Verification items for the finished model (mm, model axes). Face numbers are marked on the shaded views. A direction names the side the tool comes from. Give positions to 0.01 mm unless a question says otherwise; leave off trailing zeros. Write each loop counter-clockwise with the first axis right and the second up, starting at its lowest first coordinate (ties: lowest second). Pieces come first, ordered by that corner, then holes. Notation, with made-up numbers: (71, 51) -> (101, 51) arc R27 ccw to (101, 82) -> close; hole circle Ø4 at (62.25, 4.25). An arc over 180 degrees is marked (long way). Write item = value, one per line.
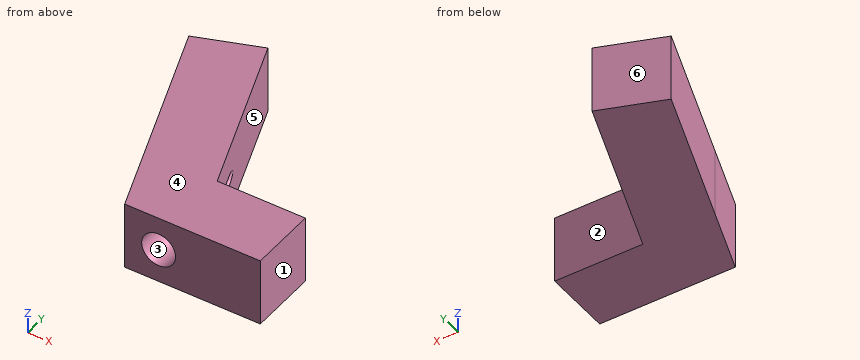
from build123d import *

# Parameters (mm, degrees)
BOSS_EXTRUDE1_DEPTH = 25.4
SKETCH3_R           = 6.35
CUT_EXTRUDE1_DEPTH  = 15.875
SKETCH4_R           = 2.0955
CUT_EXTRUDE2_DEPTH  = 98.893788925


with BuildPart() as part:
    # Sketch1 → Boss-Extrude1 (new body)
    with BuildSketch(Plane.XY):
        Polygon((0, 0), (-19.950187023, 54.81268836), (3.918005545, 63.5), (27.030115421, 0), (60.04484395, 0), (60.04484395, -25.4), (9.24484395, -25.4), align=None)
    extrude(amount=BOSS_EXTRUDE1_DEPTH)

    # Sketch3 → Cut-Extrude1 (cut)
    with BuildSketch(Plane.XZ.offset(25.4)):
        with Locations(Location((21.94484395, 12.7, 0), (0, 0, 270))):
            Circle(SKETCH3_R)
    extrude(amount=-CUT_EXTRUDE1_DEPTH, mode=Mode.SUBTRACT)

    # Sketch4 → Cut-Extrude2 (cut, through all)
    with BuildSketch(Plane.XZ.offset(9.525)):
        with Locations(Location((21.94484395, 12.7, 0), (0, 0, 270))):
            Circle(SKETCH4_R)
    extrude(amount=-CUT_EXTRUDE2_DEPTH, mode=Mode.SUBTRACT)


solid = part.part
Item 1: Set-up check for the marked faces 1 and 2: record each of +Z, -Z, +X, -X, +Y, -Y from which the full face is reachable in a straight line by a thin tool's end or side.
Response values:
face_1 = +Z, -Z, +X, +Y, -Y
face_2 = +Z, -Z, +X, +Y
Item 2: Sectioned sample at B-B on z = 20.75. Record the cut outline in (x, y).
Response values:
outline = (-19.95, 54.81) -> (9.24, -25.4) -> (60.04, -25.4) -> (60.04, 0) -> (27.03, 0) -> (3.92, 63.5) -> close
Item 3: Sectioned sample at D-D on x = 49.5. Record the cut outline in (y, z), then the cut area to 3 significant figures.
Response values:
outline = (-25.4, 0) -> (0, 0) -> (0, 25.4) -> (-25.4, 25.4) -> close
area = 645 mm^2
Item 4: Go/stop test with flat-tipped pins: P1, Ø10, axis at x = 21.94, z = 12.7, coming from the -Y side (3 decimals); P2, Ø2, axis at y = 14.5, z = 6.5, coming from the +X side; P3, Ø5, axis at x = 4, z = 22.5, coming from the +Y side. Record where each tip stops, or that it passes through.
Response values:
P1 = -9.525
P2 = 22.12
P3 = 63.5
Item 5: Sectioned sample at A-A on z = 11.75. Record the cut outline in (x, y) (3 decimals).
Response values:
outline = (-19.95, 54.813) -> (9.245, -25.4) -> (15.666, -25.4) -> (15.666, -9.525) -> (20.077, -9.525) -> (20.077, 19.103) -> (3.918, 63.5) -> close; (23.813, -9.525) -> (28.223, -9.525) -> (28.223, -25.4) -> (60.045, -25.4) -> (60.045, 0) -> (27.03, 0) -> (23.813, 8.84) -> close
Item 6: Sectioned sample at C-C on x = 17.5. Record the cut outline in (y, z) (3 decimals).
Response values:
outline = (-25.4, 0) -> (26.184, 0) -> (26.184, 25.4) -> (-25.4, 25.4) -> (-25.4, 17.235) -> (-9.525, 17.235) -> (-9.525, 8.165) -> (-25.4, 8.165) -> close
Item 7: Mould release check, pull along X, two halves, no side actions. Record for the marked faces 3, 4, 5 and 6: +X half, -X half, draft (parallel to the pull), parting line (faces both ways), or undercut.
Response values:
face_3 = undercut
face_4 = draft
face_5 = +X half
face_6 = -X half
Item 8: Material ranges on line 1 (Y direction, x = 39, z = 21.5); line 2 (X direction, y = -18.5, z = 7.5); line 3 (X direction, y = -19, z = 12.7), recorded low to high.
Response values:
line_1 = -25.4 to 0
line_2 = 6.73 to 18.3, 25.59 to 60.04
line_3 = 6.92 to 15.59, 28.29 to 60.04
